```python
from build123d import *

# Parameters (mm, degrees)
SKETCH1_R           = 41.3
BOSS_EXTRUDE1_DEPTH = 800
BOSS_EXTRUDE2_DEPTH = 3
CIRPATTERN1_COUNT   = 6


with BuildPart() as part:
    # Sketch1 → Boss-Extrude1 (new body)
    with BuildSketch(Plane.XY):
        Circle(SKETCH1_R)
    extrude(amount=BOSS_EXTRUDE1_DEPTH)

    # Sketch2 → Revolve1 (revolve)
    with BuildSketch(Plane(origin=(0, 0, 0), x_dir=(0, 0, -1), z_dir=(1, 0, 0))):
        with BuildLine():
            Line((-800, 0), (-1000, 0))
            ThreePointArc((-1000, 0), (-902.109855058, 30.867215778), (-800, 41.3))
            Line((-800, 41.3), (-800, 0))
        make_face()
    revolve(axis=Axis((0, 0, 800), (0, 0, 1)))

    # Sketch3 → Boss-Extrude2 (add, symmetric)
    with BuildSketch(Plane(origin=(0, 0, 0), x_dir=(1, 0, 0), z_dir=(0, 1, 0))):
        Polygon((41.3, -140), (101.3, -50), (101.3, -20), (41.3, 0), (0, 0), (0, -140), align=None)
    boss_extrude2 = extrude(amount=BOSS_EXTRUDE2_DEPTH, both=True)

    # CirPattern1: Boss-Extrude2 ×6 about axis
    cirpattern1_axis = Axis((0, 0, 0), (0, 0, 1))
    for i in range(1, CIRPATTERN1_COUNT):
        add(boss_extrude2.rotate(cirpattern1_axis, i * 360 / CIRPATTERN1_COUNT))


solid = part.part
```
Build history of the part. All positions in model axes, mm. A direction names the side the tool comes from. Coordinates: 2 decimals unless noted, no trailing zeros. Order: outer loops, then holes, each group sorted by start corner. A loop starts at its lowest first (then second) coordinate and runs counter-clockwise, first axis right, second up.
Item 1: Drill centre lines: L1, parallel to X at y = 1.5, z = 811.5; L2, parallel to X at y = 37, z = 372.5; L3, parallel to Y at x = 19, z = 761. Where is each one in solid material? Low to high.
Filled in:
L1: x = -41.14 to 41.14
L2: x = -18.35 to 18.35
L3: y = -36.67 to 36.67
Item 2: Drop flat-ended pins along their axis: pin 1 Ø0.8 at (x, y) = (22, 35.5) entering from +Z; pin 2 Ø6 at (y, z) = (-15, 605.5) entering from +X; pin 3 Ø1 at (y, z) = (-2, 231) entering from +X; pin 4 Ø1.5 at (x, y) = (33.5, -68) entering from +Z. Give the stop position or say it passes through.
Filled in:
pin 1: stops at z = 139.93
pin 2: stops at x = 39.52
pin 3: stops at x = 41.27
pin 4: passes through
Item 3: Tool access for faces 4 (the flat face through (34.7, 54.1, 53.5)), 5 (the flat face through (-34.7, -54.1, 53.5)), 6 (the flat face through (29.475, 57.052, 53.464)): list every direction of +Z, -Z, +X, -X, +Y, -Y with a clear straight run to the whole face (end or side of a thin tool).
Filled in:
face 4: +Z, -Z, +X
face 5: +Z, -Z, -X
face 6: +Z, -Z, +Y
Item 4: Saw through at D-D on x = -67. List the corners of the cut face in (y, z).
Filled in:
outline: (-3, 8.57) - (3, 8.57) - (3, 101.45) - (-3, 101.45) - close
Item 5: Saw through at B-B on z = 564. List the corners of the cut face in (x, y), then the cut area to 3 significant figures.
Filled in:
outline: circle Ø82.6 at (0, 0)
area: 5,360 mm2
Item 6: Saw through at C-C on x = 32.5. State how many separate pieces and enclosed holes the cut face has, then the cut area to 3 significant figures.
Filled in:
separate pieces: 3
enclosed holes: 0
area: 46,800 mm2
Item 7: Mould opens along X. For faces 1 (the flat face through (-71.72, -0.04, 10.14)), 2 (the flat face through (71.72, 0.04, 10.14)), 3 (the flat face through (-29.475, -57.052, 53.464)) say: released by +X, released by -X, zero draft, split by the parting line, or undercut.
Filled in:
face 1: released by -X
face 2: released by +X
face 3: undercut
Item 8: Saw through at A-A on y = -61.5. List the corners of the cut face in (x, z), then the cut area to 3 significant figures.
Filled in:
outline: (-38.97, 10.48) - (-32.04, 9.33) - (-32.04, 98.03) - (-38.97, 92.83) - close; (32.04, 9.33) - (38.97, 10.48) - (38.97, 92.83) - (32.04, 98.03) - close
area: 1,190 mm2
